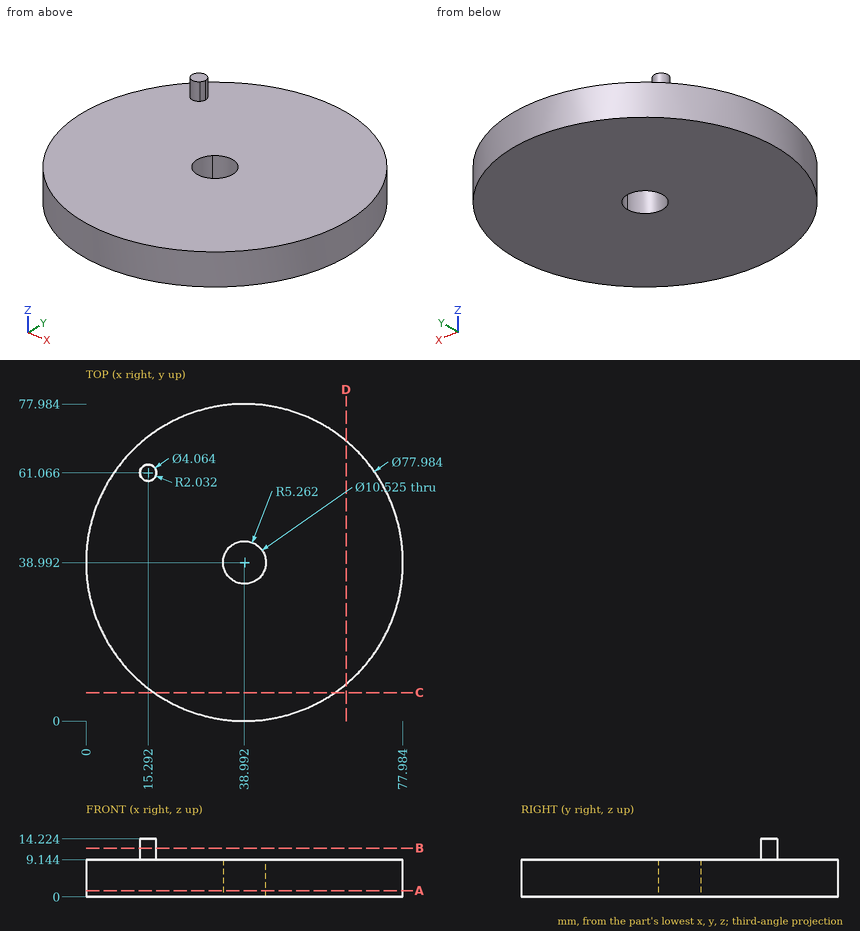
Can you work these out from the drawing? Everything is in mm from the part's minimum corner. Give positions to 0.01 mm unless a question says otherwise; leave off trailing zeros. Order: outer loops, then holes, each group sorted by start corner. A loop starts at its lowest first (then second) coordinate and runs counter-clockwise, first axis right, second up. Notation, with made-up numbers: M -13,81.5 L 29,81.5 A13 cw 29,88.5 Z; hole C 2.25,-5 d9. An arc over 180 degrees is marked long. Use a Markdown table: item, result. Add a question column.
1. Suppose I cut it at B-B (z = 12). List the corners of the cut face in (x, y) for me (1 decimal), and give its area (3 significant figures).
2. Suppose I cut it at C-C (y = 7). List the corners of the cut face in (x, z) for me (1 decimal), and give its area (3 significant figures).
3. Suppose I cut it at D-D (x = 64). List the corners of the cut face in (y, z) for me (1 decimal), and give its area (3 significant figures).
4. Suppose I cut it at A-A (z = 1.5). List the corners of the cut face in (x, y) for me (1 decimal), and give its area (3 significant figures).
5. For pin 1 Ø2 at (x, z) = (19.5, 9.5) entering from -Y; pin 2 Ø2 at (y, z) = (19.5, 10) entering from +X (1 decimal); pin 3 Ø8 at (x, z) = (56.5, 2) entering from -Y (1 decimal), each with a flat end and sliding along its axis, tell me the tip position at first contact or that it passes through.
6. I need wall thicknesses on probe 1 along Z at (x, y) = (48.5, 47) (1 decimal); probe 2 along X at (y, z) = (42.5, 3.25) (1 decimal); probe 3 along Y at (x, z) = (42, 1.25) (1 decimal). Which ranges of each line are inside material? Lowest first, please. Write a range as from..to.
Results list:
| question | item | result |
|---|---|---|
| 1 | outline | M 16.8,59.7 A2 ccw 17.3,61.1 A2 ccw long Z |
| 1 | area | 13.0 mm² |
| 2 | outline | M 16.7,0 L 61.3,0 L 61.3,9.1 L 16.7,9.1 Z |
| 2 | area | 408 mm² |
| 3 | outline | M 9.1,0 L 68.9,0 L 68.9,9.1 L 9.1,9.1 Z |
| 3 | area | 547 mm² |
| 4 | outline | C 39,39 d78; hole C 39,39 d10.5 |
| 4 | area | 4,690 mm² |
| 5 | pin 1 | stops at y = 4.7 |
| 5 | pin 2 | stops at x = 73.1 |
| 5 | pin 3 | stops at y = 2.4 |
| 6 | probe 1 | z = 0..9.1 |
| 6 | probe 2 | x = 0.2..35.1, 42.9..77.8 |
| 6 | probe 3 | y = 0.1..34.7, 43.3..77.9 |
